Autodesk Inventor part; units mm, degrees
ref_plane "Work Plane1" through (17.5, 0, 6) normal (0, 0, 1) x (1, 0, 0)
ref_plane "YZ Plane" through (0, 0, 0) normal (1, 0, 0) x (0, 1, 0)
ref_plane "XZ Plane" through (0, 0, 0) normal (0, 1, 0) x (-1, 0, 0)
sketch "Skizze1" plane through (0, 0, 0) normal (0, 0, 1) x (1, 0, 0)
  line L0 (-4, 0) -> (-4, 10)
  line L1 (-4, 10) -> (0, 10)
  line L2 (0, 10) -> (0, 6)
  line L3 (0, 6) -> (35, 6)
  line L4 (35, 6) -> (35, 0)
  line L5 (-4, 0) -> (35, 0)
  line L6 (-4, 0) -> (17, 0)
  line L7 (0, -0.98) -> (0, 3.08)
  circle A0 centre (29.5, 0) radius 1.6
  dimension "d0" = 12
  dimension "d1" = 20
  dimension "d2" = 4
  dimension "d3" = 35
  dimension "d5" = 5.5
  dimension "d6" = 3.2
revolve "Körper" add sketch "Skizze1" angle 360 about axis through (-4, 0, 0) along (1, 0, 0) picked at (29.9216, 0.9202) contours L0 L1 L2 L3 L4 L5 A0 | A0 L5
extrude "Bohrung" cut sketch "Skizze1" along normal through all both and the other way through all contours A0 L5 | L5 A0
chamfer "Fase1" distance 1.6 angle 45 1 edges at (-4, -10, 0) measured on face at (-2.6667, 9.9676, -0.8047)
chamfer "Fase2" distance 3 angle 30 1 edges at (35, -6, 0) measured on face at (21.4513, 2.8362, -5.2873)
ref_plane "Work Plane1" through (17.5, 0, 6) normal (0, 0, 1) x (1, 0, 0)
equation "\"d0\" = NND"
equation "\"d1\" = KOD"
equation "\"d2\" = KOH"
equation "\"d3\" = NLG"
equation "\"d5\" = DIST"
equation "\"d6\" = BOR"
equation "\"d7\" = NND"
equation "\"d9\" = PHH2"
equation "\"d10\" = FAWI2"
equation "\"d16\" = PHH2"
equation "\"d11\" = PHH1"
equation "\"d12\" = FAWI1"
equation "\"d17\" = PHH1"
equation "\"PHH1\" = 3"
equation "\"PHH2\" = 1.6"
equation "\"KOD\" = 20"
equation "\"KOH\" = 4"
equation "\"NND\" = 12"
equation "\"FAWI1\" = 30deg"
equation "\"FAWI2\" = 45deg"
equation "\"DIST\" = 5.5"
equation "\"BOR\" = 3.2"
equation "\"NLG\" = 35"
properties part number "IS 6863 - B12 x 35" material "Stahl, weich"
Read the model definition and answer for the solid it produces. Units are mm, in the model's axes. A direction names the side the tool comes from. Coordinates: 2 decimals unless noted, no trailing zeros. Write each loop counter-clockwise with the first axis right and the second up, starting at its lowest first coordinate (ties: lowest second). Pieces come first, ordered by that corner, then holes. Notation, with made-up numbers: (-27, 43.25) -> (-17, 43.25) arc R11 ccw to (-17, 63.25) -> close; hole circle Ø1 at (7.5, 49). An arc over 180 degrees is marked (long way). Return JSON: item names as keys, results as strings.
1. Each of these flat-tipped pins is pushed along its axis until it touches: P1, Ø3, axis at x = 5.5, y = -5.5, coming from the +Z side; P2, Ø3, axis at x = 2, y = 6.5, coming from the +Z side; P3, Ø2.5, axis at x = 29.5, y = 0, coming from the -Z side; P4, Ø3, axis at x = 18.5, y = -2, coming from the +Z side. Where does it stop, or does it pass through?
Found:
{"P1": "z = 4.47", "P2": "z = 3.32", "P3": "through", "P4": "z = 5.98"}
2. A cutting plane is placed at A-A (y = 0). Determine the outline of the cut face in (x, z).
Found:
{"outline": "(-4, -8.4) -> (-2.4, -10) -> (0, -10) -> (0, -6) -> (27.9, -6) -> (27.9, 6) -> (0, 6) -> (0, 10) -> (-2.4, 10) -> (-4, 8.4) -> close; (31.1, -6) -> (32, -6) -> (35, -4.27) -> (35, 4.27) -> (32, 6) -> (31.1, 6) -> close"}
3. Find the intervals of material crossed by line 1 along X through (y, z) = (0, 2.25); line 2 along Y through (x, z) = (29.5, -0.25); line 3 along Z through (x, y) = (12.5, 0), in increasing order. Write a range as from..to.
Found:
{"line 1": "-4..27.9, 31.1..35", "line 2": "-5.99..-1.6, 1.6..5.99", "line 3": "-6..6"}
4. A cutting plane is placed at D-D (x = 30). Determine the outline of the cut face in (y, z).
Found:
{"outline": "(-1.52, -5.8) -> (-1.52, 5.8) arc R6 ccw to start; (1.52, -5.8) arc R6 ccw to (1.52, 5.8) -> close"}
5. Determine the mould class of faces 3 (the face through (27.9, 0.07, 0.08)), 4 (the face through (-4, 0, 0)), 5 (the face through (-1.18, -2.17, -9.76)), 6 (the face through (34.812, 4.174, -1.315)) for opening direction X: pulls with the +X half, pulls with the -X half, needs draft (parallel to the pull), parting line crosses it, or undercut.
Found:
{"face 3": "undercut", "face 4": "pulls with the -X half", "face 5": "needs draft", "face 6": "pulls with the +X half"}
6. A cutting plane is placed at B-B (z = 0). Determine the outline of the cut face in (x, y), and give its area (3 significant figures).
Found:
{"outline": "(-4, -8.4) -> (-2.4, -10) -> (0, -10) -> (0, -6) -> (32, -6) -> (35, -4.27) -> (35, 4.27) -> (32, 6) -> (0, 6) -> (0, 10) -> (-2.4, 10) -> (-4, 8.4) -> close; hole circle Ø3.2 at (29.5, 0)", "area": "484 mm2"}
7. A tool of negligible diameter and unlimited length cuts with its end or side. For faces 1 (the face through (35, 0, 0)), 2 (the face through (16.224, -1.301, -5.857)), from which of +Z, -Z, +X, -X, +Y, -Y can it reach the whole face along a straight path? Write none if from no direction.
Found:
{"face 1": "+Z, -Z, +X, +Y, -Y", "face 2": "+X"}
8. A cutting plane is placed at C-C (x = 21). Determine the outline of the cut face in (y, z), and give its area (3 significant figures).
Found:
{"outline": "circle Ø12 at (0, 0)", "area": "113 mm2"}
